```python
from build123d import *

# Parameters (mm, degrees)
SKETCH1_W           = 15.24
SKETCH1_H           = 15.24
BOSS_EXTRUDE1_DEPTH = 3.81
BOSS_EXTRUDE2_DEPTH = 1.6002
SKETCH3_W           = 15.24
SKETCH3_H           = 15.24
BOSS_EXTRUDE3_DEPTH = 3.81
SKETCH4_W           = 4.318
SKETCH4_H           = 4.318
CUT_EXTRUDE1_DEPTH  = 15.182414746
SKETCH5_R           = 1.778
CUT_EXTRUDE2_DEPTH  = 15.182414746
FILLET1_R           = 1.016


with BuildPart() as part:
    # Sketch1 → Boss-Extrude1 (new body)
    with BuildSketch(Plane(origin=(0, 0, 0), x_dir=(1, 0, 0), z_dir=(0, 1, 0))):
        Rectangle(SKETCH1_W, SKETCH1_H)
    extrude(amount=BOSS_EXTRUDE1_DEPTH)

    # Sketch2 → Boss-Extrude2 (add)
    with BuildSketch(Plane(origin=(0, 3.81, 0), x_dir=(1, 0, 0), z_dir=(0, 1, 0))):
        Polygon((-7.62, 7.62), (-7.62, 1.27), (1.27, 1.27), (1.27, -7.62), (7.62, -7.62), (7.62, 7.62), align=None)
    extrude(amount=BOSS_EXTRUDE2_DEPTH)

    # Sketch3 → Boss-Extrude3 (add)
    with BuildSketch(Plane(origin=(0, 5.4102, 0), x_dir=(1, 0, 0), z_dir=(0, 1, 0))):
        Rectangle(SKETCH3_W, SKETCH3_H)
    extrude(amount=BOSS_EXTRUDE3_DEPTH)

    # Sketch4 → Cut-Extrude1 (cut, through all)
    with BuildSketch(Plane(origin=(0, 9.2202, 0), x_dir=(1, 0, 0), z_dir=(0, 1, 0))):
        with Locations((-5.461, -5.461)):
            Rectangle(SKETCH4_W, SKETCH4_H)
    extrude(amount=-CUT_EXTRUDE1_DEPTH, mode=Mode.SUBTRACT)

    # Sketch5 → Cut-Extrude2 (cut, through all)
    with BuildSketch(Plane(origin=(0, 9.2202, 0), x_dir=(1, 0, 0), z_dir=(0, 1, 0))):
        with Locations(Location((4.445, 4.445, 0), (0, 0, 270))):
            Circle(SKETCH5_R)
    extrude(amount=-CUT_EXTRUDE2_DEPTH, mode=Mode.SUBTRACT)

    # Fillet1
    fillet1_edges = [part.edges().sort_by_distance(p)[0] for p in [
        (7.62, 9.2202, 0),
        (0, 9.2202, -7.62),
        (-7.62, 9.2202, -2.159),
        (2.159, 9.2202, 7.62),
        (-3.302, 9.2202, 5.461),
        (-5.461, 9.2202, 3.302),
    ]]
    fillet(fillet1_edges, radius=FILLET1_R)


solid = part.part
```
The listing builds one solid part. Answer for the finished solid, in the listing's coordinates (mm). A direction names the side the tool comes from. Give positions to 0.01 mm unless a question says otherwise; leave off trailing zeros. Loops run counter-clockwise (first coordinate to the right, second up) from the corner with the lowest first, then second, coordinate; pieces in that order, holes last. Notation, with made-up numbers: (27.25, -38.75) - (84.25, -38.75) arc R22 ccw to (84.25, -21.75) - close; hole circle Ø1 at (57.5, 50). An arc over 180 degrees is marked (long way). Answer as CSV lines item,"result". Start each with the question number.
Item 1: For faces 1 (the face through (7.314, 8.93, -0.107)), 2 (the face through (1.27, 5, 3)), 3 (the face through (-3.302, 7, 5)), 4 (the face through (-4.916, 8.93, 2.996)), determine the directions among +Z, -Z, +X, -X, +Y, -Y from which every point of the face is accessible in a straight line to the end or side of a thin tool.
Item 2: The mould has two halves that part along Y. Classify faces 5 (the face through (0, 9.22, 0)), 6 (the face through (7.62, 4, 0)), 7 (the face through (-3, 5, -1.27)): +Y half, -Y half, draft (parallel to the pull), parting line (faces both ways), or undercut.
Item 3: A cutting plane is placed at A-A on z = -5.5. Determine the outline of the cut face in (x, y), then the cut area to 3 significant figures.
Item 4: A cutting plane is placed at B-B on x = -3.75. Determine the outline of the cut face in (y, z), then the cut area to 3 significant figures.
Item 5: Find the intervals of material crossed by line 1 (X direction, y = 1.25, z = -4.5); line 2 (Y direction, x = 0.75, z = 0); line 3 (Z direction, x = -5, y = 1.5), in increasing order. Write a range as from..to.
Item 6: A cutting plane is placed at D-D on z = 0. Determine the outline of the cut face in (x, y).
Item 7: Each of these flat-tipped pins is pushed along its axis until it touches: pin 1 (1.8 mm diameter, centred on y = 4.5, z = 4.5, fed in from -X); pin 2 (0.8 mm diameter, centred on x = -5.5, y = 7, fed in from +Z). Where does it stop, or does it pass through?
Item 8: A cutting plane is placed at C-C on y = 4.5. Determine the outline of the cut face in (x, z) (3 decimals).
Found:
1,face 1,"+Z, -Z, +X, +Y"
1,face 2,"+Z, -X"
1,face 3,"+Z, -X, +Y, -Y"
1,face 4,"+Z, -X, +Y"
2,face 5,"+Y half"
2,face 6,"draft"
2,face 7,"undercut"
3,outline,"(-7.62, 0) - (3.01, 0) - (3.01, 9.22) - (-6.6, 9.22) arc R1.02 ccw to (-7.62, 8.2) - close; (5.88, 0) - (7.62, 0) - (7.62, 8.2) arc R1.02 ccw to (6.6, 9.22) - (5.88, 9.22) - close"
3,area,"114 mm^2"
4,outline,"(0, -7.62) - (8.2, -7.62) arc R1.02 ccw to (9.22, -6.6) - (9.22, 2.29) arc R1.02 ccw to (8.2, 3.3) - (5.41, 3.3) - (5.41, -1.27) - (3.81, -1.27) - (3.81, 3.3) - (0, 3.3) - close"
4,area,"92.9 mm^2"
5,line 1,"x = -7.62..2.67, 6.22..7.62"
5,line 2,"y = 0..3.81, 5.41..9.22"
5,line 3,"z = -7.62..3.3"
6,outline,"(-7.62, 0) - (7.62, 0) - (7.62, 8.2) arc R1.02 ccw to (6.6, 9.22) - (-6.6, 9.22) arc R1.02 ccw to (-7.62, 8.2) - (-7.62, 5.41) - (1.27, 5.41) - (1.27, 3.81) - (-7.62, 3.81) - close"
7,pin 1,"stops at x = -3.3"
7,pin 2,"stops at z = 3.3"
8,outline,"(-7.62, -7.62) - (7.62, -7.62) - (7.62, 7.62) - (1.27, 7.62) - (1.27, -1.27) - (-7.62, -1.27) - close; hole circle Ø3.556 at (4.445, -4.445)"
